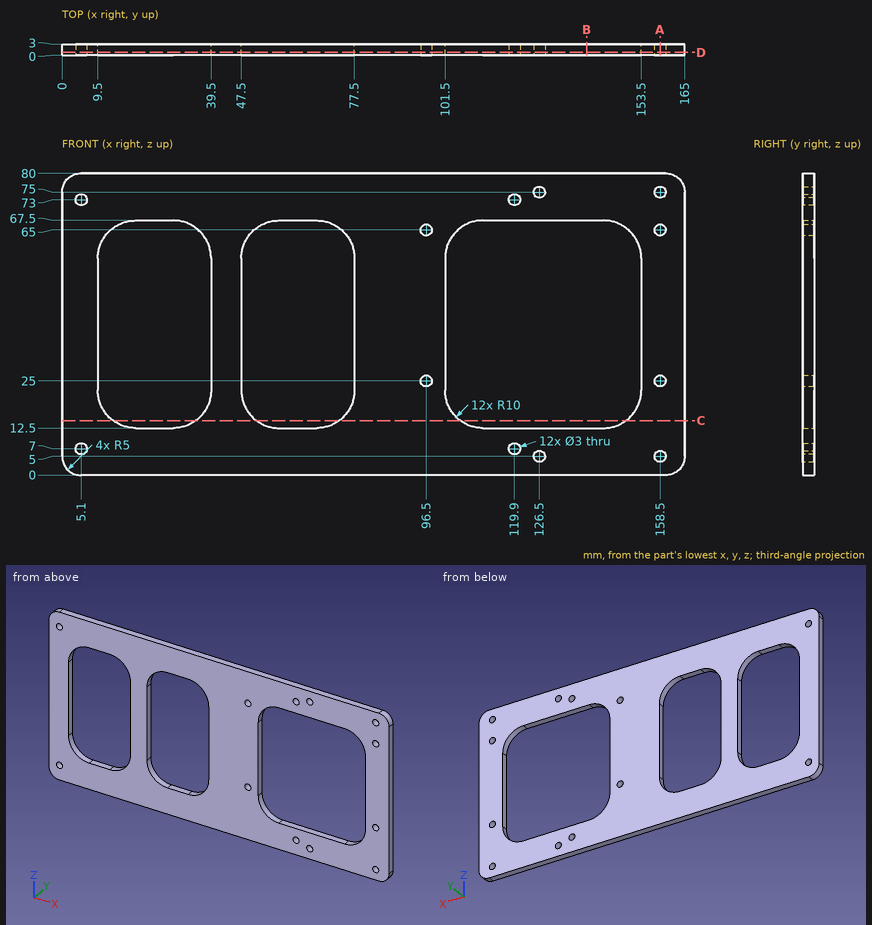
For this review, use the dimensioned drawing (mm, ordinates from the lowest corner) and the shaded views. Give positions to 0.01 mm unless a question says otherwise; leave off trailing zeros. Order: outer loops, then holes, each group sorted by start corner. A loop starts at its lowest first (then second) coordinate and runs counter-clockwise, first axis right, second up.
1) Take a section at C-C (z = 14.5). Give the boundary of the cut face in (x, y), then the cut area to 3 significant figures.
2) Insertion check: pin 1 (2.5 mm diameter, centred on x = 158.5, z = 25, fed in from +Y); pin 2 (4 mm diameter, centred on x = 96.5, z = 25, fed in from -Y). Each pin has a flat end and moves straight along its axis. Give the tip position at first contact, or say it passes through.
3) Take a section at D-D (y = 0.75). State how many separate pieces and enclosed holes the cut face has, then the cut area to 3 significant figures.
4) Wall thickness on line 1 (X direction, y = 2.85, z = 39); line 2 (Z direction, x = 119.9, y = 0.9); line 3 (Z direction, x = 158.5, y = 2): over which ranges is each line inside the solid? List them lowest first.
5) Take a section at B-B (x = 139). Give the boundary of the cut face in (y, z).
6) Take a section at A-A (x = 158.5). Give the boundary of the cut face in (y, z), then the cut area to 3 significant figures.
Derived:
1. outline: (0, 0) - (13.5, 0) - (13.5, 3) - (0, 3) - close; (35.5, 0) - (51.5, 0) - (51.5, 3) - (35.5, 3) - close; (73.5, 0) - (105.5, 0) - (105.5, 3) - (73.5, 3) - close; (149.5, 0) - (165, 0) - (165, 3) - (149.5, 3) - close
1. area: 231 mm2
2. pin 1: passes through
2. pin 2: stops at y = 0
3. separate pieces: 1
3. enclosed holes: 15
3. area: 7,190 mm2
4. line 1: x = 0 to 9.5, 39.5 to 47.5, 77.5 to 101.5, 153.5 to 165
4. line 2: z = 0 to 5.5, 8.5 to 12.5, 67.5 to 71.5, 74.5 to 80
4. line 3: z = 0 to 3.5, 6.5 to 23.5, 26.5 to 63.5, 66.5 to 73.5, 76.5 to 80
5. outline: (0, 0) - (3, 0) - (3, 12.5) - (0, 12.5) - close; (0, 67.5) - (3, 67.5) - (3, 80) - (0, 80) - close
6. outline: (0, 0) - (3, 0) - (3, 3.5) - (0, 3.5) - close; (0, 6.5) - (3, 6.5) - (3, 23.5) - (0, 23.5) - close; (0, 26.5) - (3, 26.5) - (3, 63.5) - (0, 63.5) - close; (0, 66.5) - (3, 66.5) - (3, 73.5) - (0, 73.5) - close; (0, 76.5) - (3, 76.5) - (3, 80) - (0, 80) - close
6. area: 204 mm2
